Verification items for the finished model (mm, model axes). Face numbers are marked on the shaded views. A direction names the side the tool comes from. Round coordinates to 2 decimals unless told otherwise and drop trailing zeros. Write each loop counter-clockwise with the first axis right and the second up, starting at its lowest first coordinate (ties: lowest second). Pieces come first, ordered by that corner, then holes. Notation, with made-up numbers: M -29.75,38 L -7.75,38 A15 cw -7.75,48 Z; hole C 35,78 d8. An arc over 180 degrees is marked long. One line per item, written item: value. Start each with the question number.
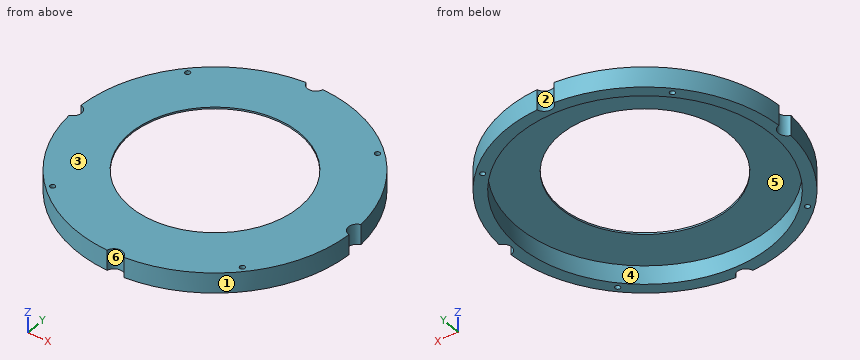
from build123d import *
from build123d.topology import SkipClean

# Parameters (mm, degrees)
SKETCH1_R           = 82
SKETCH1_R_2         = 50
BOSS_EXTRUDE1_DEPTH = 1
BOSS_EXTRUDE3_START = 11
SKETCH3_R           = 82
SKETCH3_R_2         = 75
BOSS_EXTRUDE3_DEPTH = 11
SKETCH4_R           = 5
CUT_EXTRUDE1_DEPTH  = 117.584733134
CIRPATTERN1_COUNT   = 4
SKETCH5_R           = 1.5
CUT_EXTRUDE2_DEPTH  = 117.381356407
CIRPATTERN2_COUNT   = 4


with BuildPart() as part:
    # Sketch1 → Boss-Extrude1 (new body)
    with BuildSketch(Plane.XY):
        Circle(SKETCH1_R)
        Circle(SKETCH1_R_2, mode=Mode.SUBTRACT)
    extrude(amount=BOSS_EXTRUDE1_DEPTH)

    # Sketch3 → Boss-Extrude3 (add)
    with BuildSketch(Plane(origin=(0, 0, 0), x_dir=(-1, 0, 0), z_dir=(0, 0, -1)).offset(BOSS_EXTRUDE3_START)):
        Circle(SKETCH3_R)
        Circle(SKETCH3_R_2, mode=Mode.SUBTRACT)
    extrude(amount=-BOSS_EXTRUDE3_DEPTH)

    # Sketch4 → Cut-Extrude1 (cut, through all)
    with SkipClean():  # the faces are left unmerged after this step: merging them gives an invalid solid
        with BuildSketch(Plane.XY.offset(1)):
            with Locations((0, 83)):
                Circle(SKETCH4_R)
        cut_extrude1 = extrude(amount=-CUT_EXTRUDE1_DEPTH, mode=Mode.SUBTRACT)

    # CirPattern1: Cut-Extrude1 ×4 about axis
    cirpattern1_axis = Axis((0, 0, 0), (0, 0, 1))
    for i in range(1, CIRPATTERN1_COUNT):
        add(cut_extrude1.rotate(cirpattern1_axis, i * 360 / CIRPATTERN1_COUNT), mode=Mode.SUBTRACT)

    # Sketch5 → Cut-Extrude2 (cut, through all)
    with BuildSketch(Plane(origin=(0, 0, -11), x_dir=(-1, 0, 0), z_dir=(0, 0, -1))):
        with Locations((55.507882323, 55.507882323)):
            Circle(SKETCH5_R)
    cut_extrude2 = extrude(amount=-CUT_EXTRUDE2_DEPTH, mode=Mode.SUBTRACT)

    # CirPattern2: Cut-Extrude2 ×4 about axis
    cirpattern2_axis = Axis((0, 0, 0), (0, 0, 1))
    for i in range(1, CIRPATTERN2_COUNT):
        add(cut_extrude2.rotate(cirpattern2_axis, i * 360 / CIRPATTERN2_COUNT), mode=Mode.SUBTRACT)


solid = part.part
1) Thickness scan on line 1 (Y direction, x = -54.5, z = -9.5); line 2 (Z direction, x = -48, y = -35); line 3 (X direction, y = -19.5, z = -9.75). Record the ranges inside material, lowest first.
2) Gauge pin test, flat ends, axial feed: pin 1 Ø2 at (y, z) = (6, -7.5) entering from +X; pin 2 Ø4 at (y, z) = (32.5, -1) entering from -X; pin 3 Ø4 at (y, z) = (18.5, -4) entering from +X. Record the tip position at first contact, or that the pin passes through.
3) Mould release check, pull along X, two halves, no side actions. Record for the marked faces 1, 2, 3 and 4: pulls with the +X half, pulls with the -X half, needs draft (parallel to the pull), parting line crosses it, or undercut.
4) Cross-section at D-D (y = 65). Record the boundary of the cut face in (x, z).
5) Cross-section at C-C (z = -8). Record the boundary of the cut face in (x, y), then the cut area to 3 significant figures.
6) Cross-section at A-A (x = 0). Record the boundary of the cut face in (y, z), then the cut area to 3 significant figures.
7) Access from +Z, -Z, +X, -X, +Y, -Y to the whole of each face (thin tool, end or side, straight path). Record for the marked faces 5 and 6.
Results below:
1. line 1: y = -61.27 to -56.62, -54.4 to -51.52, 51.52 to 54.4, 56.62 to 61.27
1. line 2: z = 0 to 1
1. line 3: x = -79.65 to -72.42, 72.42 to 79.65
2. pin 1: stops at x = 81.85
2. pin 2: stops at x = -76.12
2. pin 3: stops at x = 80.32
3. face 1: pulls with the +X half
3. face 2: undercut
3. face 3: needs draft
3. face 4: undercut
4. outline: M -49.99,-11 L -37.42,-11 L -37.42,0 L 37.42,0 L 37.42,-11 L 49.99,-11 L 49.99,1 L -49.99,1 Z
5. outline: M -81.86,-4.87 A82 ccw -4.87,-81.86 A5 cw 4.87,-81.86 A82 ccw 81.86,-4.87 A5 cw 81.86,4.87 A82 ccw 4.87,81.86 A5 cw -4.87,81.86 A82 ccw -81.86,4.87 A5 cw Z; hole C 0,0 d150; hole C -55.51,-55.51 d3; hole C -55.51,55.51 d3; hole C 55.51,-55.51 d3; hole C 55.51,55.51 d3
5. area: 3,310 mm²
6. outline: M -78,-11 L -75,-11 L -75,0 L -50,0 L -50,1 L -78,1 Z; M 50,0 L 75,0 L 75,-11 L 78,-11 L 78,1 L 50,1 Z
6. area: 122 mm²
7. face 5: -Z
7. face 6: +Z, -Z, -Y
